```python
from build123d import *

# Parameters (mm, degrees)
SKETCH1_W           = 12.7
SKETCH1_H           = 88.9
SKETCH1_R           = 2.31
BOSS_EXTRUDE1_DEPTH = 1.5875
SKETCH3_W           = 2.038660884
SKETCH3_H           = 88.935455435
BOSS_EXTRUDE3_DEPTH = 10


with BuildPart() as part:
    # Sketch1 → Boss-Extrude1 (new body)
    with BuildSketch(Plane(origin=(0, 0, 0), x_dir=(1, 0, 0), z_dir=(0, 1, 0))):
        with Locations((6.35, 57.087542426)):
            Rectangle(SKETCH1_W, SKETCH1_H)
        with Locations(Location((6.293214881, 95.187542426, 0), (0, 0, 270))):
            Circle(SKETCH1_R, mode=Mode.SUBTRACT)
        with Locations(Location((6.293214881, 31.537542426, 0), (0, 0, 270))):
            Circle(SKETCH1_R, mode=Mode.SUBTRACT)
    extrude(amount=BOSS_EXTRUDE1_DEPTH)

    # Sketch3 → Boss-Extrude3 (add)
    with BuildSketch(Plane(origin=(0, 0, 0), x_dir=(-1, 0, 0), z_dir=(0, -1, 0))):
        with Locations((-0.999274051, 57.069814709)):
            Rectangle(SKETCH3_W, SKETCH3_H)
    extrude(amount=BOSS_EXTRUDE3_DEPTH)


solid = part.part
```
Source: CAD feature listing. Evaluate the final solid. Frame: model axes, mm. A direction names the side the tool comes from. Round coordinates to 2 decimals unless told otherwise and drop trailing zeros. Loops run counter-clockwise (first coordinate to the right, second up) from the corner with the lowest first, then second, coordinate; pieces in that order, holes last. Notation, with made-up numbers: M 70.25,26.5 L 115.25,26.5 A10 ccw 115.25,30.5 Z; hole C 60.5,-10 d7. An arc over 180 degrees is marked long. Use a Markdown table: item, result. Add a question column.
1. Contact query for flat-ended pins moving along their axis: pin 1 (1.7 mm diameter, centred on x = 3, y = 1, fed in from +Z); pin 2 (0.8 mm diameter, centred on y = 1, z = -37, fed in from -X); pin 3 (5.5 mm diameter, centred on x = 6.29, z = -31.54, fed in from +Y); pin 4 (1 mm diameter, centred on x = 5, z = -22, fed in from -Y). Output: stop coordinate, or through.
2. Set-up query: faces 5 (the flat face through (7, 0, -58)), 6 (the flat face through (12.7, 1, -56)). Return all of +Z, -Z, +X, -X, +Y, -Y with unobstructed straight access to the full face (end or side cutting, diameter ignored); none if empty.
3. Cut plane D-D, the plane y = -9. Output: boundary loops of the cut face in (x, z).
4. Ray query, line 1 along Y through (x, z) = (6, -35); line 2 along X through (y, z) = (-3.25, -48); line 3 along Z through (x, y) = (10.5, 0.25). Return the intervals inside material, ascending. Write a range as [from, to].
5. Cut plane C-C, the plane x = 2.75. Output: boundary loops of the cut face in (y, z).
6. Pull-direction query (X, two-part tool) for faces 1 (the cylindrical face through (8.241, 0.783, -30.296)), 2 (the flat face through (1.7, -1.6, -101.538)), 3 (the flat face through (0, 1, -56)), 4 (the flat face through (2.019, -5, -56)); classes: +X half, -X half, draft (parallel to the pull), parting line (faces both ways), or undercut.
Solution:
| question | item | result |
|---|---|---|
| 1 | pin 1 | stops at z = -12.64 |
| 1 | pin 2 | stops at x = 0 |
| 1 | pin 3 | stops at y = 1.59 |
| 1 | pin 4 | stops at y = 0 |
| 2 | face 5 | +Z, -Z, +X, -Y |
| 2 | face 6 | +Z, -Z, +X, +Y, -Y |
| 3 | outline | M -0.02,-101.54 L 2.02,-101.54 L 2.02,-12.6 L -0.02,-12.6 Z |
| 4 | line 1 | y = [0, 1.59] |
| 4 | line 2 | x = [-0.02, 2.02] |
| 4 | line 3 | z = [-101.54, -12.64] |
| 5 | outline | M 0,-101.54 L 1.59,-101.54 L 1.59,-12.64 L 0,-12.64 Z |
| 6 | face 1 | undercut |
| 6 | face 2 | draft |
| 6 | face 3 | -X half |
| 6 | face 4 | +X half |
